from build123d import *

# Parameters (mm, degrees)
SKETCH_1_W                  = 27
SKETCH_1_H                  = 15
EXTRUDE_1_DEPTH             = 1
SKETCH_2_R                  = 2.425
CUT_EXTRUDE_1_DEPTH         = 16.475787541
EXTRUDE_2_DEPTH             = 15
SKETCH_6_W                  = 1.5
SKETCH_6_H                  = 2
EXTRUDE_3_DEPTH             = 4
SKETCH_7_R                  = 1.35
CUT_EXTRUDE_3_DEPTH         = 1.5
FILLET_1_R                  = 3
CHAMFER_1_SIZE              = 1
CUT_EXTRUDE_4_REACH         = 39.101
SKETCH_8_R                  = 2
SKETCH_9_W                  = 21.5
SKETCH_9_H                  = 30
EXTRUDE_4_DEPTH             = 1
EXTRUDE_5_REACH             = 54.216
EXTRUDE_5_DIRECTION_2_REACH = 54.216
FILLET_2_R                  = 10
FILLET_3_R                  = 0.5


# Some blends are built 0.0001 mm under size
with BuildPart() as part:
    # 草图1 → 凸台-拉伸1 (new body)
    with BuildSketch(Plane.XY):
        Rectangle(SKETCH_1_W, SKETCH_1_H)
    extrude(amount=EXTRUDE_1_DEPTH)

    # 草图2 → 切除-拉伸1 (cut, through all)
    with BuildSketch(Plane.XY.offset(1)):
        with Locations((0, 4.025)):
            Circle(SKETCH_2_R)
        with Locations((0, -4.025)):
            Circle(SKETCH_2_R)
        with Locations((8.05, 4.025)):
            Circle(SKETCH_2_R)
        with Locations((8.05, -4.025)):
            Circle(SKETCH_2_R)
        with Locations((-8.05, 4.025)):
            Circle(SKETCH_2_R)
        with Locations((-8.05, -4.025)):
            Circle(SKETCH_2_R)
    extrude(amount=-CUT_EXTRUDE_1_DEPTH, mode=Mode.SUBTRACT)

    # 草图3 → 凸台-拉伸2 (add)
    with BuildSketch(Plane.XZ.offset(7.5)):
        Polygon((13.5, 0), (19, 0), (19, -28.5), (-4.5, -28.5), (-4.5, -30), (20.5, -30), (20.5, 1), (13.5, 1), align=None)
    extrude(amount=-EXTRUDE_2_DEPTH)

    # 草图6 → 凸台-拉伸3 (add, symmetric)
    with BuildSketch(Plane(origin=(0, 0, 0), x_dir=(1, 0, 0), z_dir=(0, 1, 0))):
        Polygon((19, 0), (19, 5), (14, 0), align=None)
        Polygon((19, 28.5), (14, 28.5), (19, 23.5), align=None)
        with Locations((18.25, 20)):
            Rectangle(SKETCH_6_W, SKETCH_6_H)
    extrude(amount=EXTRUDE_3_DEPTH, both=True)

    # 草图7 → 切除-拉伸3 (cut)
    with BuildSketch(Plane(origin=(0, 0, -30), x_dir=(-1, 0, 0), z_dir=(0, 0, -1))):
        with BuildLine():
            ThreePointArc((4.5, 0), (3.401301202, -2.946379157), (0.641711051, -4.454010207))
            Line((0.641711051, -4.454010207), (-20.5, -7.5))
            Line((-20.5, -7.5), (4.5, -7.5))
            Line((4.5, -7.5), (4.5, 0))
        make_face()
        with BuildLine():
            Line((-20.5, 7.5), (0.641711051, 4.454010207))
            ThreePointArc((0.641711051, 4.454010207), (3.401301202, 2.946379157), (4.5, 0))
            Line((4.5, 0), (4.5, 7.5))
            Line((4.5, 7.5), (-20.5, 7.5))
        make_face()
        Circle(SKETCH_7_R)
    extrude(amount=-CUT_EXTRUDE_3_DEPTH, mode=Mode.SUBTRACT)

    # 圆角1
    # the kernel refuses this fillet: 3 mm, written as the material it adds along each edge
    with BuildSketch(Plane(origin=(19, -3.5, -28.5), x_dir=(-1, 0, 0), z_dir=(0, 1, 0))) as fillet_1_piece_1_section:
        with BuildLine():
            CenterArc((FILLET_1_R, FILLET_1_R), FILLET_1_R, 180, 90)
            Line((0, FILLET_1_R), (0, 0))
            Line((0, 0), (FILLET_1_R, 0))
        make_face()
    fillet_1_piece_1 = extrude(amount=18.283887658, mode=Mode.PRIVATE)
    fillet_1_piece_1 = split(fillet_1_piece_1, bisect_by=Plane(origin=(18.119115161, 7.156974268, -27.821481802), z_dir=(0.1426024558755584, -0.9897800460598605, 0)), keep=Keep.TOP, mode=Mode.PRIVATE)
    add(fillet_1_piece_1)
    with BuildSketch(Plane(origin=(19, -3.5, 0), x_dir=(0, 0, -1), z_dir=(0, 1, 0)), Plane(origin=(19, -7.5, 0), x_dir=(0, 0, -1), z_dir=(0, 1, 0))) as fillet_1_piece_2:
        with BuildLine():
            CenterArc((FILLET_1_R, FILLET_1_R), FILLET_1_R, 180, 90)
            Line((0, FILLET_1_R), (0, 0))
            Line((0, 0), (FILLET_1_R, 0))
        make_face()
    extrude(amount=11)
    with BuildSketch(Plane(origin=(19, -14.783887658, -28.5), x_dir=(-1, 0, 0), z_dir=(0, 1, 0))) as fillet_1_piece_3_section:
        with BuildLine():
            CenterArc((FILLET_1_R, FILLET_1_R), FILLET_1_R, 180, 90)
            Line((0, FILLET_1_R), (0, 0))
            Line((0, 0), (FILLET_1_R, 0))
        make_face()
    fillet_1_piece_3 = extrude(amount=18.283887658, mode=Mode.PRIVATE)
    fillet_1_piece_3 = split(fillet_1_piece_3, bisect_by=Plane(origin=(18.119115161, -7.156974268, -27.821481802), z_dir=(0.1426024558755584, 0.9897800460598605, 0)), keep=Keep.TOP, mode=Mode.PRIVATE)
    add(fillet_1_piece_3)
    # the kernel refuses this fillet: 3 mm, written as the material it takes off along each edge
    with BuildSketch(Plane(origin=(20.5, -15, 1), x_dir=(0, 0, -1), z_dir=(0, 1, 0))) as fillet_1_2_piece_1:
        with BuildLine():
            CenterArc((FILLET_1_R, FILLET_1_R), FILLET_1_R, 180, 90)
            Line((0, FILLET_1_R), (0, 0))
            Line((0, 0), (FILLET_1_R, 0))
        make_face()
    extrude(amount=30, mode=Mode.SUBTRACT)
    with BuildSketch(Plane(origin=(20.5, -15, -30), x_dir=(0, 0, 1), z_dir=(0, 1, 0))) as fillet_1_2_piece_2:
        with BuildLine():
            CenterArc((FILLET_1_R, -FILLET_1_R), FILLET_1_R, 90, 90)
            Line((0, -FILLET_1_R), (0, 0))
            Line((0, 0), (FILLET_1_R, 0))
        make_face()
    extrude(amount=30, mode=Mode.SUBTRACT)

    # 倒角1
    chamfer_1_edges = [part.edges().sort_by_distance(p)[0] for p in [
        (-13.5, 0, 0),
    ]]
    chamfer(chamfer_1_edges, length=CHAMFER_1_SIZE - 0.0001)  # a hair under: the kernel refuses the full size

    # 草图8 → 切除-拉伸4 (cut, up to next)
    with BuildSketch(Plane(origin=(0, 0, 0), x_dir=(-1, 0, 0), z_dir=(0, 0, -1)), mode=Mode.PRIVATE) as cut_extrude_4_sk1:
        Circle(SKETCH_8_R)
    cut_extrude_4_tool1 = extrude(cut_extrude_4_sk1.sketch, amount=-CUT_EXTRUDE_4_REACH, mode=Mode.PRIVATE) & part.part
    add(cut_extrude_4_tool1.solids().sort_by_distance((0, 0, 0))[0], mode=Mode.SUBTRACT)

    # 草图9 → 凸台-拉伸4 (add)
    with BuildSketch(Plane.XY.offset(1)):
        with Locations((0, 22.5)):
            Rectangle(SKETCH_9_W, SKETCH_9_H)
    extrude(amount=-EXTRUDE_4_DEPTH)

    # 凸台-拉伸5: up to this face of the body (flat: up to its plane)
    extrude_5_end = Plane(part.part.faces().sort_by_distance((-10.75, 22.5, 0.5))[0])
    # 草图10 → 凸台-拉伸5 (add, up to the picked face)
    with BuildSketch(Plane(origin=(0, 0, 0), x_dir=(0, 0, -1), z_dir=(1, 0, 0)), mode=Mode.PRIVATE) as extrude_5_sk1:
        with BuildLine():
            Line((-1, 37.5), (0, 37.5))
            Line((0, 37.5), (18.572123903, 59.633395384))
            Line((18.572123903, 59.633395384), (17.80607946, 60.276182993))
            Line((17.80607946, 60.276182993), (-0.766044443, 38.14278761))
            ThreePointArc((-0.766044443, 38.14278761), (-0.939692621, 37.842020143), (-1, 37.5))
        make_face()
    extrude_5_tool1 = split(extrude(extrude_5_sk1.sketch, amount=-EXTRUDE_5_REACH, mode=Mode.PRIVATE), bisect_by=extrude_5_end, keep=Keep.BOTH, mode=Mode.PRIVATE)
    add(extrude_5_tool1.solids().sort_by(Axis((0, 48.754818, -8.789436), (-1, 0, 0)))[0])

    # 凸台-拉伸5 direction 2: up to this face of the body (flat: up to its plane)
    extrude_5_direction_2_end = Plane(part.part.faces().sort_by_distance((10.75, 22.5, 0.5))[0])
    # 草图10 → 凸台-拉伸5 direction 2 (add, up to the picked face)
    with BuildSketch(Plane(origin=(0, 0, 0), x_dir=(0, 0, -1), z_dir=(1, 0, 0)), mode=Mode.PRIVATE) as extrude_5_direction_2_sk1:
        with BuildLine():
            Line((-1, 37.5), (0, 37.5))
            Line((0, 37.5), (18.572123903, 59.633395384))
            Line((18.572123903, 59.633395384), (17.80607946, 60.276182993))
            Line((17.80607946, 60.276182993), (-0.766044443, 38.14278761))
            ThreePointArc((-0.766044443, 38.14278761), (-0.939692621, 37.842020143), (-1, 37.5))
        make_face()
    extrude_5_direction_2_tool1 = split(extrude(extrude_5_direction_2_sk1.sketch, amount=EXTRUDE_5_DIRECTION_2_REACH, mode=Mode.PRIVATE), bisect_by=extrude_5_direction_2_end, keep=Keep.BOTH, mode=Mode.PRIVATE)
    add(extrude_5_direction_2_tool1.solids().sort_by(Axis((0, 48.754818, -8.789436), (1, 0, 0)))[0])

    # 圆角2
    fillet_2_edges = [part.edges().sort_by_distance(p)[0] for p in [
        (0, 37.5, 0),
    ]]
    fillet(fillet_2_edges, radius=FILLET_2_R)

    # 圆角3
    fillet_3_edges = [part.edges().sort_by_distance(p)[0] for p in [
        (0, 60.276182993, -17.80607946),
        (0, 59.633395384, -18.572123903),
    ]]
    fillet(fillet_3_edges, radius=FILLET_3_R - 0.0001)  # a hair under: the kernel refuses the full size


solid = part.part
Input: part model. Units: mm. Frame: model coordinates. A direction names the side the tool comes from. Give positions to 0.01 mm unless a question says otherwise; leave off trailing zeros. Loops run counter-clockwise (first coordinate to the right, second up) from the corner with the lowest first, then second, coordinate; pieces in that order, holes last. Notation, with made-up numbers: (49.25, -22) -> (68.25, -22) arc R21 cw to (68.25, -1) -> close; hole circle Ø7 at (68, 39). An arc over 180 degrees is marked (long way). Answer as a JSON object with one key per item and string values. Group by question number.
Item 1: Pin query (flat end, axial travel): P1, Ø1.5, axis at x = 12.5, z = -4, coming from the +Y side; P2, Ø1.6, axis at x = 18.5, y = 0, coming from the -Z side; P3, Ø1.5, axis at x = -4.5, y = 34.5, coming from the -Z side; P4, Ø3, axis at x = 8.05, y = 4.025, coming from the +Z side. Return the tip coordinate at first contact, or that it passes through.
Item 2: Cut plane C-C, the plane z = -6.5. Return the cut outline in (x, y).
Item 3: Reachability of faces 4 (the flat face through (10.75, 40, -1)), 5 (the cylindrical face through (18.1, 5.73, -0.86)), 6 (the flat face through (17, -4, -2)), 7 (the flat face through (16.5, -0.1, -26)) from +Z, -Z, +X, -X, +Y, -Y: full face, straight path, thin tool, end or side. Return the list, or none.
Item 4: Pull-direction query (Y, two-part tool) for faces 1 (the flat face through (17, 0, -3)), 2 (the cylindrical face through (7.52, -6.39, 0.51)), 3 (the flat face through (17, -4, -27)); classes: released by +Y, released by -Y, zero draft, split by the parting line, or undercut.
Item 5: Line query: probe 1 along Y at (x, z) = (-8.05, 0.7); probe 2 along Z at (x, y) = (7.5, 21); probe 3 along X at (y, z) = (6.5, -9.5). Output: solid intervals per line, ascending.
Item 6: Cut plane A-A, the plane x = -8.05. State how many separate pieces and enclosed holes the cut face has, and give its area (3 significant figures).
Item 7: Cut plane D-D, the plane y = 9.5. Return the cut outline in (x, z).
Checks:
{
 "1": {"P1": "passes through", "P2": "stops at z = -29.99", "P3": "stops at z = -0.1", "P4": "stops at z = -28.5"},
 "2": {"outline": "(-10.75, 45.25) -> (10.75, 45.25) -> (10.75, 46.8) -> (-10.75, 46.8) -> close; (19, -7.5) -> (20.5, -7.5) -> (20.5, 7.5) -> (19, 7.5) -> close"},
 "3": {"face 4": "+Z, -Z, +X, +Y", "face 5": "-X, +Y", "face 6": "-X, -Y", "face 7": "-X, +Y, -Y"},
 "4": {"face 1": "zero draft", "face 2": "undercut", "face 3": "released by -Y"},
 "5": {"probe 1": "y = -7.5 to -6.45, -1.6 to 1.6, 6.45 to 38.22", "probe 2": "z = 0 to 1", "probe 3": "x = 19 to 20.5"},
 "6": {"separate pieces": "3", "enclosed holes": "0", "area": "65.9 mm²"},
 "7": {"outline": "(-10.75, 0) -> (10.75, 0) -> (10.75, 1) -> (-10.75, 1) -> close"}
}
